Verification items for the finished model (mm, model axes). Face numbers are marked on the shaded views. A direction names the side the tool comes from. Round coordinates to 2 decimals unless told otherwise and drop trailing zeros. Write each loop counter-clockwise with the first axis right and the second up, starting at its lowest first coordinate (ties: lowest second). Pieces come first, ordered by that corner, then holes. Notation, with made-up numbers: M 60,44.25 L 99,44.25 A19 ccw 99,78.25 Z; hole C 49,71 d5. An arc over 180 degrees is marked long. Answer in a Markdown table with one row per item. Add a question column.
1. Sectioned sample at C-C on x = 44.5. Record the cut outline in (y, z), plus the area to 3 significant figures.
2. Set-up check for the marked faces 1, 2 and 3: record each of +Z, -Z, +X, -X, +Y, -Y from which the full face is reachable in a straight line by a thin tool's end or side.
3. Sectioned sample at A-A on y = 3.5. Record the cut outline in (x, z).
4. Draft check along Y on the marked faces 4, 5 and 6. Enter one of: pulls with the +Y half, pulls with the -Y half, needs draft (parallel to the pull), parting line crosses it, or undercut.
5. Sectioned sample at D-D on y = 16.45. Record the cut outline in (x, z), plus the area to 3 significant figures.
6. Material ranges on probe 1 along X at (y, z) = (1, 5); probe 2 along X at (y, z) = (8.25, 2.05); probe 3 along Y at (x, z) = (44.5, 1.65), recorded low to high.
7. Sectioned sample at B-B on z = 3.85. Record the cut outline in (x, y), plus the area to 3 significant figures.
8. Go/stop test with flat-tipped pins: pin 1 Ø2 at (x, z) = (30.5, 1.5) entering from -Y; pin 2 Ø1.6 at (x, z) = (15, 3) entering from +Y; pin 3 Ø1.2 at (y, z) = (20, 3) entering from -X. Record where each tip stops, or that it passes through.
```python
from build123d import *

# Parameters (mm, degrees)
MODEL_R             = 1.2
MODEL_W             = 5.350001156
MODEL_H             = 13.50000035
BOSS_EXTRUDE1_DEPTH = 5.35


with BuildPart() as part:
    # Model → Boss-Extrude1 (new body)
    with BuildSketch(Plane.XY):
        with BuildLine():
            Line((3.000000026, 15.449999832), (25.000000373, 15.449999832))
            ThreePointArc((25.000000373, 15.449999832), (27.121321034, 16.328679314), (28.000000864, 18.449999832))
            Line((28.000000864, 18.449999832), (28.000000864, 22.45000054))
            ThreePointArc((28.000000864, 22.45000054), (28.878680036, 24.571320398), (30.999999493, 25.450000539))
            Line((30.999999493, 25.450000539), (50.000000745, 25.450000539))
            Line((50.000000745, 25.450000539), (50.000000745, 0))
            Line((50.000000745, 0), (39.000000805, 0))
            Line((39.000000805, 0), (39.000000805, 5.350000225))
            Line((39.000000805, 5.350000225), (10.99999994, 5.350000225))
            Line((10.99999994, 5.350000225), (10.99999994, 0))
            Line((10.99999994, 0), (0, 0))
            Line((0, 0), (0, 12.449999832))
            ThreePointArc((0, 12.449999832), (0.878679666, 14.571320184), (3.000000026, 15.449999832))
        make_face()
        with Locations((44.5, 16.45)):
            Circle(MODEL_R, mode=Mode.SUBTRACT)
        with Locations((34.175001085, 12.20000023)):
            Rectangle(MODEL_W, MODEL_H, mode=Mode.SUBTRACT)
    extrude(amount=BOSS_EXTRUDE1_DEPTH)


solid = part.part
```
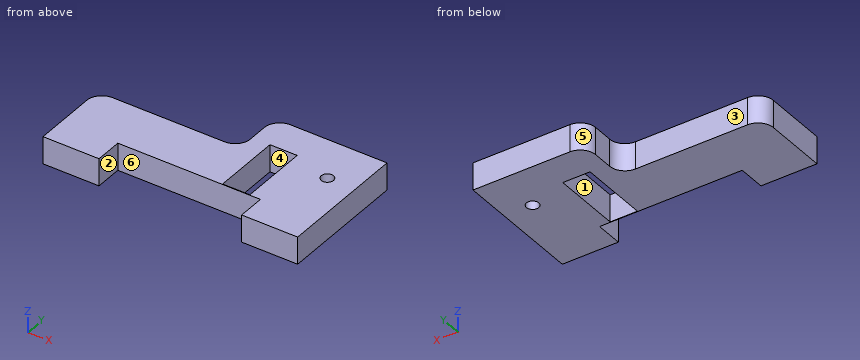
Geometry check:
| question | item | result |
|---|---|---|
| 1 | outline | M 0,0 L 15.25,0 L 15.25,5.35 L 0,5.35 Z; M 17.65,0 L 25.45,0 L 25.45,5.35 L 17.65,5.35 Z |
| 1 | area | 123 mm2 |
| 2 | face 1 | +Z, -Z |
| 2 | face 2 | +Z, -Z, -Y |
| 2 | face 3 | +Z, -Z, -X, +Y |
| 3 | outline | M 0,0 L 11,0 L 11,5.35 L 0,5.35 Z; M 39,0 L 50,0 L 50,5.35 L 39,5.35 Z |
| 4 | face 4 | undercut |
| 4 | face 5 | pulls with the +Y half |
| 4 | face 6 | pulls with the -Y half |
| 5 | outline | M 27.24,0 L 31.5,0 L 31.5,5.35 L 27.24,5.35 Z; M 36.85,0 L 43.3,0 L 43.3,5.35 L 36.85,5.35 Z; M 45.7,0 L 50,0 L 50,5.35 L 45.7,5.35 Z |
| 5 | area | 80.3 mm2 |
| 6 | probe 1 | x = 0 to 11, 39 to 50 |
| 6 | probe 2 | x = 0 to 31.5, 36.85 to 50 |
| 6 | probe 3 | y = 0 to 15.25, 17.65 to 25.45 |
| 7 | outline | M 0,0 L 11,0 L 11,5.35 L 39,5.35 L 39,0 L 50,0 L 50,25.45 L 31,25.45 A3 ccw 28,22.45 L 28,18.45 A3 cw 25,15.45 L 3,15.45 A3 ccw 0,12.45 Z; hole M 31.5,5.45 L 36.85,5.45 L 36.85,18.95 L 31.5,18.95 Z; hole C 44.5,16.45 d2.4 |
| 7 | area | 764 mm2 |
| 8 | pin 1 | stops at y = 5.35 |
| 8 | pin 2 | stops at y = 15.45 |
| 8 | pin 3 | stops at x = 28 |
